Verification items for the finished model (mm, model axes). A direction names the side the tool comes from. Coordinates: 2 decimals unless noted, no trailing zeros. Order: outer loops, then holes, each group sorted by start corner. A loop starts at its lowest first (then second) coordinate and runs counter-clockwise, first axis right, second up. Notation, with made-up numbers: (56.5, 21) -> (88.5, 21) arc R23 cw to (88.5, 52) -> close; hole circle Ø4 at (64, -32.75). An arc over 180 degrees is marked (long way). Answer as CSV lines item,"result".
```python
from build123d import *

# Parameters (mm, degrees)
F1_DEPTH = 7.4
F0_W     = 31.5
F0_H     = 12
F2_DEPTH = 2
F4_DEPTH = 25
F5_R     = 0.5
F6_R     = 0.5


# Not quite as in the source:
# - a feature names something its author has since deleted; it is built from what else it names


with BuildPart() as f1:
    # F0 (on Top) → F1 (new body)
    with BuildSketch(Plane.XY):
        Polygon((15.75, -9), (15.75, -6), (-15.75, -6), (-15.75, -9), (-15.75, -9.970754717), (-13.55, -9.970754717), (-13.55, -9), (13.55, -9), (13.55, -9.970754717), (15.75, -9.970754717), align=None)
    extrude(amount=F1_DEPTH)



with BuildPart() as f1b:
    # F0 (on Top) → F1, piece 2 (new body)
    with BuildSketch(Plane.XY):
        Polygon((13.55, 9.970754717), (13.55, 9), (-13.55, 9), (-13.55, 9.970754717), (-15.75, 9.970754717), (-15.75, 9), (-15.75, 6), (15.75, 6), (15.75, 9), (15.75, 9.970754717), align=None)
    extrude(amount=F1_DEPTH)


with BuildPart() as f1_1:
    add(f1.part)

    add(f1b.part)  # F2 merges F1b
    # F0 (on Top) → F2 (join)
    with BuildSketch(Plane.XY):
        Rectangle(F0_W, F0_H)
    extrude(amount=F2_DEPTH)

    # F3 (on face) → F4 (cut)
    with BuildSketch(Plane.XY):
        Polygon((-0.5079215625, -1.4132374693), (-10.6910164902, -5.2925117274), (-0.5079215625, -5.2925117274), align=None)
        Polygon((10.6910164902, -5.2925117274), (0.5079215625, -1.4132374693), (0.5079215625, -5.2925117274), align=None)
        Polygon((1.7789258686, -0.5523047257), (14.6478014067, -5.4547335021), (14.6478014067, -0.5523047257), (14.6478014067, 0.5523047257), (14.6478014067, 5.4547335021), (1.7789258686, 0.5523047257), align=None)
        Polygon((0.5079215625, 1.4132374693), (10.6910164902, 5.2925117274), (0.5079215625, 5.2925117274), align=None)
        Polygon((-0.5079215625, 5.2925117274), (-10.6910164902, 5.2925117274), (-0.5079215625, 1.4132374693), align=None)
        with BuildLine():
            Line((-9.222632274, 6), (9.222632274, 6))
            Line((9.222632274, 6), (9.222632274, 6.5901111811))
            ThreePointArc((9.222632274, 6.5901111811), (9.513632274, 6.8811111811), (9.804632274, 6.5901111811))
            Line((9.804632274, 6.5901111811), (13.0790583789, 6.5901111811))
            Line((13.0790583789, 6.5901111811), (13.7675590813, 6.5901111811))
            Line((13.7675590813, 6.5901111811), (14.6781420335, 6.5901111811))
            Line((14.6781420335, 6.5901111811), (14.6781420335, 8.4549048916))
            Line((14.6781420335, 8.4549048916), (13.7675590813, 8.4549048916))
            Line((13.7675590813, 8.4549048916), (13.0790583789, 8.4549048916))
            Line((13.0790583789, 8.4549048916), (7.4084047228, 8.4549048916))
            Line((7.4084047228, 8.4549048916), (6.8271243945, 8.4549048916))
            Line((6.8271243945, 8.4549048916), (-6.8271243945, 8.4549048916))
            Line((-6.8271243945, 8.4549048916), (-7.4084047228, 8.4549048916))
            Line((-7.4084047228, 8.4549048916), (-13.0790583789, 8.4549048916))
            Line((-13.0790583789, 8.4549048916), (-13.7675590813, 8.4549048916))
            Line((-13.7675590813, 8.4549048916), (-14.6781420335, 8.4549048916))
            Line((-14.6781420335, 8.4549048916), (-14.6781420335, 6.5901111811))
            Line((-14.6781420335, 6.5901111811), (-13.7675590813, 6.5901111811))
            Line((-13.7675590813, 6.5901111811), (-13.0790583789, 6.5901111811))
            Line((-13.0790583789, 6.5901111811), (-9.804632274, 6.5901111811))
            ThreePointArc((-9.804632274, 6.5901111811), (-9.513632274, 6.8811111811), (-9.222632274, 6.5901111811))
            Line((-9.222632274, 6.5901111811), (-9.222632274, 6))
        make_face()
        Polygon((-14.6478014067, 5.4547335021), (-14.6478014067, 0.5523047257), (-14.6478014067, -0.5523047257), (-14.6478014067, -5.4547335021), (-1.7789258686, -0.5523047257), (-1.7789258686, 0.5523047257), align=None)
        with BuildLine():
            Line((9.222632274, -6.5901111811), (9.222632274, -6))
            Line((9.222632274, -6), (-9.222632274, -6))
            Line((-9.222632274, -6), (-9.222632274, -6.5901111811))
            ThreePointArc((-9.222632274, -6.5901111811), (-9.513632274, -6.8811111811), (-9.804632274, -6.5901111811))
            Line((-9.804632274, -6.5901111811), (-13.0790583789, -6.5901111811))
            Line((-13.0790583789, -6.5901111811), (-13.7675590813, -6.5901111811))
            Line((-13.7675590813, -6.5901111811), (-14.6781420335, -6.5901111811))
            Line((-14.6781420335, -6.5901111811), (-14.6781420335, -8.4549048916))
            Line((-14.6781420335, -8.4549048916), (-13.7675590813, -8.4549048916))
            Line((-13.7675590813, -8.4549048916), (-13.0790583789, -8.4549048916))
            Line((-13.0790583789, -8.4549048916), (-7.4084047228, -8.4549048916))
            Line((-7.4084047228, -8.4549048916), (-6.8271243945, -8.4549048916))
            Line((-6.8271243945, -8.4549048916), (6.8271243945, -8.4549048916))
            Line((6.8271243945, -8.4549048916), (7.4084047228, -8.4549048916))
            Line((7.4084047228, -8.4549048916), (13.0790583789, -8.4549048916))
            Line((13.0790583789, -8.4549048916), (13.7675590813, -8.4549048916))
            Line((13.7675590813, -8.4549048916), (14.6781420335, -8.4549048916))
            Line((14.6781420335, -8.4549048916), (14.6781420335, -6.5901111811))
            Line((14.6781420335, -6.5901111811), (13.7675590813, -6.5901111811))
            Line((13.7675590813, -6.5901111811), (13.0790583789, -6.5901111811))
            Line((13.0790583789, -6.5901111811), (9.804632274, -6.5901111811))
            ThreePointArc((9.804632274, -6.5901111811), (9.513632274, -6.8811111811), (9.222632274, -6.5901111811))
        make_face()
    extrude(amount=F4_DEPTH, mode=Mode.SUBTRACT)

    # F5
    f5_edges = [f1_1.edges().sort_by_distance(p)[0] for p in [
        (-15.75, 6, 4.7),
        (-15.75, -6, 4.7),
        (15.75, 6, 4.7),
        (15.75, -6, 4.7),
        (15.75, -9.970755, 3.7),
        (-15.75, -9.970755, 3.7),
        (-15.75, 9.970755, 3.7),
        (15.75, 9.970755, 3.7),
    ]]
    fillet(f5_edges, radius=F5_R)

    # F6
    f6_edges = [f1_1.edges().sort_by_distance(p)[0] for p in [
        (-9.222632, 6, 4.7),
        (9.222632, 6, 4.7),
        (9.222632, -6, 4.7),
        (-9.222632, -6, 4.7),
    ]]
    fillet(f6_edges, radius=F6_R)


solid = f1_1.part
```
Item 1: Section check B-B, the plane y = -4. Record the boundary of the cut face in (x, z).
Answer list:
outline,"(-15.75, 0) -> (-14.65, 0) -> (-14.65, 2) -> (-15.75, 2) -> close; (-10.83, 0) -> (-7.3, 0) -> (-7.3, 2) -> (-10.83, 2) -> close; (-0.51, 0) -> (0.51, 0) -> (0.51, 2) -> (-0.51, 2) -> close; (7.3, 0) -> (10.83, 0) -> (10.83, 2) -> (7.3, 2) -> close; (14.65, 0) -> (15.75, 0) -> (15.75, 2) -> (14.65, 2) -> close"
Item 2: Depth check by flat-ended pin: pin 1 Ø1.5 at (x, y) = (2, -6.5) entering from +Z; pin 2 Ø0.6 at (x, z) = (-2, 0.5) entering from -Y; pin 3 Ø1 at (x, z) = (-9, 2) entering from +Y. Enter the tip coordinate at first touch or a pass-through.
Answer list:
pin 1,"z = 2"
pin 2,"y = -9"
pin 3,"y = 9"
Item 3: Section check A-A, the plane x = -1. Record the boundary of the cut face in (y, z).
Answer list:
outline,"(-9, 0) -> (-8.45, 0) -> (-8.45, 7.4) -> (-9, 7.4) -> close; (-6, 0) -> (-5.29, 0) -> (-5.29, 2) -> (-6, 2) -> close; (-1.6, 0) -> (1.6, 0) -> (1.6, 2) -> (-1.6, 2) -> close; (5.29, 0) -> (6, 0) -> (6, 2) -> (5.29, 2) -> close; (8.45, 0) -> (9, 0) -> (9, 7.4) -> (8.45, 7.4) -> close"
Item 4: Section check C-C, the plane x = 11.5. Record the boundary of the cut face in (y, z).
Answer list:
outline,"(-9, 0) -> (-8.45, 0) -> (-8.45, 7.4) -> (-9, 7.4) -> close; (-6.59, 0) -> (-4.26, 0) -> (-4.26, 2) -> (-6, 2) -> (-6, 7.4) -> (-6.59, 7.4) -> close; (4.26, 0) -> (6.59, 0) -> (6.59, 7.4) -> (6, 7.4) -> (6, 2) -> (4.26, 2) -> close; (8.45, 0) -> (9, 0) -> (9, 7.4) -> (8.45, 7.4) -> close"
Item 5: Tool access check on faces 1 (the flat face through (-12, -6.59, 4)), 2 (the flat face through (-14, 9.971, 4)). Record the directions out of +Z, -Z, +X, -X, +Y, -Y that give a thin tool (end or side, any length) a straight path to the whole face; none if there is none.
Answer list:
face 1,"+Z, -Z"
face 2,"+Z, -Z, +X, -X, +Y"
Item 6: Thickness scan on line 1 (Y direction, x = 11, z = 3); line 2 (Y direction, x = -0.5, z = 7.25); line 3 (Y direction, x = -5, z = 1). Record the ranges inside material, lowest first.
Answer list:
line 1,"-9 to -8.45, -6.59 to -6, 6 to 6.59, 8.45 to 9"
line 2,"-9 to -8.45, 8.45 to 9"
line 3,"-9 to -8.45, -6 to -5.29, -3.12 to -1.78, 1.78 to 3.12, 5.29 to 6, 8.45 to 9"
Item 7: Section check D-D, the plane z = 1.25. Count the separate pieces of the cut face and the enclosed holes in it, plus the area to 3 significant figures.
Answer list:
separate pieces,"1"
enclosed holes,"8"
area,"211 mm2"
Item 8: Release check for a two-part mould opening along Y. For faces 3 (the flat face through (5.67, -3.38, 0.99)), 4 (the flat face through (0, 1, 0)), 5 (the flat face through (14, 9.971, 4)) record: +Y half, -Y half, draft (parallel to the pull), parting line (faces both ways), or undercut.
Answer list:
face 3,"undercut"
face 4,"draft"
face 5,"+Y half"
